from build123d import *

# Parameters (mm, degrees)
BOSS_EXTRUDE1_DEPTH = 19.05
SKETCH3_R           = 22.5
CUT_EXTRUDE1_DEPTH  = 17
FILLET1_R           = 2
FILLET2_R           = 1


with BuildPart() as part:
    # Sketch2 → Boss-Extrude1 (new body)
    with BuildSketch(Plane(origin=(0, 0, 0), x_dir=(1, 0, 0), z_dir=(0, 1, 0))):
        with BuildLine():
            Line((79.031032842, 24.025126848), (79.031032842, 15.211900093))
            ThreePointArc((79.031032842, 15.211900093), (79.61681928, 13.797686531), (81.031032842, 13.211900093))
            Line((81.031032842, 13.211900093), (92.031032842, 13.211900093))
            ThreePointArc((92.031032842, 13.211900093), (93.445246404, 13.797686531), (94.031032842, 15.211900093))
            Line((94.031032842, 15.211900093), (94.031032842, 81.211900093))
            ThreePointArc((94.031032842, 81.211900093), (93.445246404, 82.626113656), (92.031032842, 83.211900093))
            Line((92.031032842, 83.211900093), (81.031032842, 83.211900093))
            ThreePointArc((81.031032842, 83.211900093), (79.61681928, 82.626113656), (79.031032842, 81.211900093))
            Line((79.031032842, 81.211900093), (79.031032842, 72.398673338))
            ThreePointArc((79.031032842, 72.398673338), (77.728518675, 70.524236486), (75.517519329, 71.09128019))
            ThreePointArc((75.517519329, 71.09128019), (14.031032842, 48.211900093), (75.517519329, 25.332519997))
            ThreePointArc((75.517519329, 25.332519997), (77.728518675, 25.899563701), (79.031032842, 24.025126848))
        make_face()
    extrude(amount=BOSS_EXTRUDE1_DEPTH)

    # Sketch3 → Cut-Extrude1 (cut)
    with BuildSketch(Plane(origin=(0, 19.05, 0), x_dir=(1, 0, 0), z_dir=(0, 1, 0))):
        with BuildLine():
            Line((82.031032842, 16.211900093), (91.031032842, 16.211900093))
            Line((91.031032842, 16.211900093), (91.031032842, 80.211900093))
            Line((91.031032842, 80.211900093), (82.031032842, 80.211900093))
            Line((82.031032842, 80.211900093), (82.031032842, 72.398673338))
            ThreePointArc((82.031032842, 72.398673338), (78.774747423, 67.712581207), (73.247249058, 69.130190467))
            ThreePointArc((73.247249058, 69.130190467), (17.031032842, 48.211900093), (73.247249058, 27.293609719))
            ThreePointArc((73.247249058, 27.293609719), (78.774747423, 28.711218979), (82.031032842, 24.025126848))
            Line((82.031032842, 24.025126848), (82.031032842, 16.211900093))
        make_face()
        with Locations(Location((49.031032842, 48.211900093, 0), (0, 0, 270))):
            Circle(SKETCH3_R, mode=Mode.SUBTRACT)
    extrude(amount=-CUT_EXTRUDE1_DEPTH, mode=Mode.SUBTRACT)

    # Fillet1
    fillet1_edges = [part.edges().sort_by_distance(p)[0] for p in [
        (82.031032842, 10.55, -16.211900093),
        (82.031032842, 10.55, -80.211900093),
        (91.031032842, 10.55, -80.211900093),
        (91.031032842, 10.55, -16.211900093),
    ]]
    fillet(fillet1_edges, radius=FILLET1_R)

    # Fillet2
    fillet2_edges = [part.edges().sort_by_distance(p)[0] for p in [
        (82.031032842, 2.05, -21.118513471),
        (78.774747423, 2.05, -28.711218979),
        (17.031032842, 2.05, -48.211900093),
        (78.774747423, 2.05, -67.712581207),
        (91.031032842, 2.05, -48.211900093),
        (86.531032842, 2.05, -16.211900093),
        (86.531032842, 2.05, -80.211900093),
        (82.031032842, 2.05, -75.305286716),
        (82.61681928, 2.05, -79.626113656),
        (90.445246404, 2.05, -79.626113656),
        (82.61681928, 2.05, -16.797686531),
        (90.445246404, 2.05, -16.797686531),
    ]]
    fillet(fillet2_edges, radius=FILLET2_R)


solid = part.part
Read the model definition and answer for the solid it produces. Units are mm, in the model's axes. A direction names the side the tool comes from. Give positions to 0.01 mm unless a question says otherwise; leave off trailing zeros. Write each loop counter-clockwise with the first axis right and the second up, starting at its lowest first coordinate (ties: lowest second). Pieces come first, ordered by that corner, then holes. Notation, with made-up numbers: (-22, 65.25) - (30, 65.25) arc R19 ccw to (30, 90.25) - close; hole circle Ø2 at (43, -30.5). An arc over 180 degrees is marked (long way). Answer in a Markdown table with one row per item. Add a question column.
Item 1: A tool of negligible diameter and unlimited length cuts with its end or side. For faces 1 (the face through (14.05, 9.39, -49.4)), 2 (the face through (75, 19.05, -69)), 3 (the face through (79.031, 9, -77)), 4 (the face through (79.031, 9, -20)), 5 (the face through (82.031, 11, -75)), from which of +Z, -Z, +X, -X, +Y, -Y can it reach the whole face along a straight path? Write none if from no direction.
Item 2: Find the intervals of material crossed by L1, parallel to Z at x = 34, y = 14.75; L2, parallel to Z at x = 60, y = 4.5; L3, parallel to X at y = 4.5, z = -20.5, in increasing order.
Item 3: Determine the mould class of faces 6 (the face through (78.69, 11.16, -28.74)), 7 (the face through (93.46, 9.39, -82.61)), 8 (the face through (86, 9, -13.212)) for opening direction X: pulls with the +X half, pulls with the -X half, needs draft (parallel to the pull), parting line crosses it, or undercut.
Item 4: Flat-ended cylindrical pins translate along their axes: P1, Ø10, axis at x = 55, y = 12, coming from the +Z side; P2, Ø8, axis at y = 12.5, z = -70, coming from the -X side; P3, Ø7, axis at y = 7.5, z = -77, coming from the -X side. Find the tip coordinate at first contact, or state that the pin passes through.
Item 5: Section A-A, the plane y = 4.25 is taken. Write down the section's boundary in (x, z), and give its area (3 significant figures).
Recorded:
| question | item | result |
|---|---|---|
| 1 | face 1 | +Y, -Y |
| 1 | face 2 | +Z, -Z, +X, -X, +Y |
| 1 | face 3 | -Z, +Y, -Y |
| 1 | face 4 | +Z, +Y, -Y |
| 1 | face 5 | +Y |
| 2 | L1 | z = -79.82 to -76.46, -64.95 to -31.47, -19.96 to -16.6 |
| 2 | L2 | z = -81.45 to -78.27, -67.86 to -28.57, -18.15 to -14.98 |
| 2 | L3 | x = 27.65 to 33.03, 65.03 to 70.41, 79.03 to 82.03, 91.03 to 94.03 |
| 3 | face 6 | undercut |
| 3 | face 7 | pulls with the +X half |
| 3 | face 8 | needs draft |
| 4 | P1 | stops at z = -13.23 |
| 4 | P2 | stops at x = 18.89 |
| 4 | P3 | stops at x = 24.83 |
| 5 | outline | circle Ø45 at (49.03, -48.21); (75.52, -71.09) arc R2 cw to (79.03, -72.4) - (79.03, -81.21) arc R2 ccw to (81.03, -83.21) - (92.03, -83.21) arc R2 ccw to (94.03, -81.21) - (94.03, -15.21) arc R2 ccw to (92.03, -13.21) - (81.03, -13.21) arc R2 ccw to (79.03, -15.21) - (79.03, -24.03) arc R2 cw to (75.52, -25.33) arc R35 ccw (long way) to start; hole (73.25, -69.13) arc R5 cw to (82.03, -72.4) - (82.03, -78.21) arc R2 ccw to (84.03, -80.21) - (89.03, -80.21) arc R2 ccw to (91.03, -78.21) - (91.03, -18.21) arc R2 ccw to (89.03, -16.21) - (84.03, -16.21) arc R2 ccw to (82.03, -18.21) - (82.03, -24.03) arc R5 cw to (73.25, -27.29) arc R32 ccw (long way) to start |
| 5 | area | 2,460 mm2 |
